The model under review builds one solid part; all positions refer to its coordinate system, in mm. Face numbers are marked on the shaded views. A direction names the side the tool comes from. Coordinates: 2 decimals unless noted, no trailing zeros. Loops run counter-clockwise (first coordinate to the right, second up) from the corner with the lowest first, then second, coordinate; pieces in that order, holes last. Notation, with made-up numbers: M 19.25,-18 L 36.25,-18 A15 cw 36.25,7 Z; hole C 81.25,-17 d9. An arc over 180 degrees is marked long. Use CSV: the item, a comma, the result in double quotes. Start each with the question number.
1. Add section B-B, the plane z = -0.5. Write out the cut boundary in (x, y).
2. Draft analysis for pull direction Z (two halves, no side actions). For the marked faces 5, 6 and 7, state which applies: +Z half, -Z half, draft (parallel to the pull), parting line (faces both ways), or undercut.
3. Add section D-D, the plane y = 2.5. Write out the cut boundary in (x, z).
4. Add section C-C, the plane y = 13.75. Write out the cut boundary in (x, z).
5. Add section A-A, the plane x = 0. Write out the cut boundary in (y, z), then the cut area to 3 significant figures.
6. Tool access review of the marked faces 1, 2, 3 and 4: name each direction out of +Z, -Z, +X, -X, +Y, -Y from which nothing blocks a thin tool from reaching the whole face with its end or side.
7. Clearance check with flat-ended pins moving along their axes: P1, Ø1, axis at y = 21, z = 3, coming from the +X side; P2, Ø5, axis at x = 1.5, y = 19.5, coming from the +Z side; P3, Ø1, axis at y = 21, z = -1, coming from the +X side; P4, Ø4, axis at x = 0.5, z = -1, coming from the -Y side. State where each tip first meets the part, or that it passes through.
8. For L1, parallel to Z at x = 0, y = 8.75; L2, parallel to Y at x = -1, z = 3.5; L3, parallel to Z at x = 0, y = 25.5, list the stretches that pass through material, from the lowest coordinate up.
Autodesk Inventor part; units mm, degrees
ref_plane "YZ Plane" through (0, 0, 0) normal (1, 0, 0) x (0, 1, 0)
ref_plane "XZ Plane" through (0, 0, 0) normal (0, 1, 0) x (-1, 0, 0)
ref_plane "XY Plane" through (0, 0, 0) normal (0, 0, 1) x (1, 0, 0)
sketch "Sketch4" plane through (0, 0, 0) normal (0, 1, 0) x (-1, 0, 0)
  circle A0 centre (0, 0) radius 4.5
  dimension "d6" = 9
extrude "Extrusion2" add sketch "Sketch4" along normal blind 13
sketch "Sketch5" plane through (0, 13, 0) normal (0, 1, 0) x (1, 0, 0)
  circle A0 centre (0, 0) radius 2.25
  line L0 (-1.45, -1.7205) -> (-1.45, 1.7205)
  dimension "d9" = 4.5
  dimension "d10" = 3.7
extrude "Extrusion3" cut sketch "Sketch5" against normal blind 13 contours A0 L0 picked at (-0.101, 0.4724)
sketch "Sketch7" plane through (0, 13, 0) normal (0, 1, 0) x (1, 0, 0)
  line L0 (-3.58, 0) -> (-1.79, 3.1004)
  line L1 (-1.79, 3.1004) -> (1.79, 3.1004)
  line L2 (1.79, 3.1004) -> (3.58, 0)
  line L3 (3.58, 0) -> (1.79, -3.1004)
  line L4 (1.79, -3.1004) -> (-1.79, -3.1004)
  line L5 (-1.79, -3.1004) -> (-3.58, 0)
  point P0 (0, 0)
  point P1 (0, 0)
  dimension "d15" = 7.16
extrude "Extrusion5" add sketch "Sketch7" along normal blind 16.5 and the other way blind 0.5
sketch "Sketch15" plane through (-1.45, 0, 1.7205) normal (1, 0, 0) x (0, 0, -1)
  circle A0 centre (1.7748, 6.2834) radius 1
  point P0 (1.7205, 0)
  dimension "d41" = 2
extrude "Extrusion11" cut sketch "Sketch15" against normal blind 4.25
sketch "Sketch9" plane through (-1.45, 0, 1.3129) normal (1, 0, 0) x (0, 0, -1)
  circle A0 centre (1.3129, 5.7735) radius 1
  point P0 (1.3129, 0)
  dimension "d21" = 2
sketch "Sketch10" plane through (-3.75, 5.7735, 0) normal (-1, 0, 0) x (0, 0, 1)
  point P0 (0, -5.7735)
  point P1 (-0.001, 0.0019)
sketch "Sketch1" plane through (0, 0, 0) normal (0, 1, 0) x (-1, 0, 0)
  circle A0 centre (0, 0) radius 12.5
  dimension "d0" = 25
  dimension "d3" = 4
  dimension "d4" = 7
  dimension "d5" = 3.5
properties part number "As JGA To Mecanum 2_3DPrint"
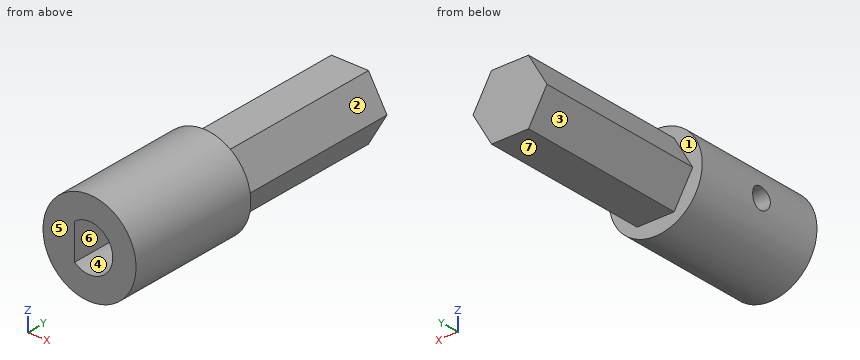
Computed:
1,outline,"M -4.47,0 L -1.45,0 L -1.45,5.39 L -4.47,5.39 Z; M -4.47,7.18 L -1.45,7.18 L -1.45,12.5 L 2.19,12.5 L 2.19,0 L 4.47,0 L 4.47,13 L 3.29,13 L 3.29,29.5 L -3.29,29.5 L -3.29,13 L -4.47,13 Z"
2,face 5,"draft"
2,face 6,"undercut"
2,face 7,"-Z half"
3,outline,"C 0,0 d9; hole M -1.45,-1.72 A2.25 ccw long -1.45,1.72 Z"
4,outline,"M -3.58,0 L -1.79,-3.1 L 1.79,-3.1 L 3.58,0 L 1.79,3.1 L -1.79,3.1 Z"
5,outline,"M 0,-4.5 L 13,-4.5 L 13,-3.1 L 29.5,-3.1 L 29.5,3.1 L 13,3.1 L 13,4.5 L 0,4.5 L 0,2.25 L 12.5,2.25 L 12.5,-2.25 L 0,-2.25 Z"
5,area,"163 mm^2"
6,face 1,"+Y"
6,face 2,"+Z, +X, +Y"
6,face 3,"-Z, -X, +Y"
6,face 4,"-Y"
7,P1,"stops at x = 2.14"
7,P2,"stops at z = 3.1"
7,P3,"stops at x = 3.29"
7,P4,"stops at y = 0"
8,L1,"z = -4.5 to -2.25, 2.25 to 4.5"
8,L2,"y = 0 to 13"
8,L3,"z = -3.1 to 3.1"
